Autodesk Inventor part; units mm, degrees
ref_plane "YZ Plane" through (0, 0, 0) normal (1, 0, 0) x (0, 1, 0)
ref_plane "XZ Plane" through (0, 0, 0) normal (0, 1, 0) x (-1, 0, 0)
ref_plane "XY Plane" through (0, 0, 0) normal (0, 0, 1) x (1, 0, 0)
sketch "Sketch1" plane through (0, 0, 0) normal (0, 0, 1) x (1, 0, 0)
  line L0 (-12.7, 12.7) -> (12.7, 12.7)
  line L1 (12.7, 12.7) -> (12.7, -12.7)
  line L2 (12.7, -12.7) -> (-12.7, -12.7)
  line L3 (-12.7, -12.7) -> (-12.7, 12.7)
  line L4 (0, 17.78) -> (0, -17.78)
  line L5 (-17.78, 0) -> (17.78, 0)
  line L6 (9.525, 9.525) -> (-9.525, 9.525)
  line L7 (-9.525, 9.525) -> (-9.525, -9.525)
  line L8 (-9.525, -9.525) -> (9.525, -9.525)
  line L9 (9.525, -9.525) -> (9.525, 9.525)
  point P0 (0, 0)
  dimension "d0" = 25.4
  dimension "d1" = 3.175
extrude "Extrusion1" add sketch "Sketch1" along normal mid plane 1502.0343 contours L0 L4 L6 L7 L5 L3 | L0 L1 L5 L9 L6 L4 | L5 L7 L8 L4 L2 L3 | L1 L2 L4 L8 L9 L5
sketch "Sketch2" plane through (12.7, 12.7, 751.0172) normal (1, 0, 0) x (0, 0, -1)
  line L0 (-300.4069, -12.7) -> (1802.4412, -12.7)
  line L1 (751.0172, -30.48) -> (751.0172, 5.08)
  circle A0 centre (12.7, -12.7) radius 3.175
  circle A1 centre (1489.3343, -12.7) radius 3.175
  point P0 (751.0172, -12.7)
  dimension "d4" = 1476.6343
  dimension "d5" = 6.35
extrude "Extrusion2" cut sketch "Sketch2" against normal up to surface (25.4 mm away)
equation "\"d2\" = Length"
equation "\"d6\" = Length"
properties part number "NTowerSupport" material "Aluminum 6061"
Input: part model. Units: mm. Frame: model coordinates. Give positions to 0.01 mm unless a question says otherwise; leave off trailing zeros. Order: outer loops, then holes, each group sorted by start corner. A loop starts at its lowest first (then second) coordinate and runs counter-clockwise, first axis right, second up. Notation, with made-up numbers: M 75,-38 L 113,-38 A16 ccw 113,-18 Z; hole C 78.25,-22.5 d3. An arc over 180 degrees is marked long. One line per question, with ' | ' between items.
1) Ray query, L1, parallel to X at y = 5.5, z = 561.5 (3 decimals); L2, parallel to Z at x = -11, y = 2. Return the intervals inside material, ascending.
Filled in:
L1: x = -12.7 to -9.525, 9.525 to 12.7 | L2: z = -751.02 to -740.78, -735.85 to 735.85, 740.78 to 751.02
2) Section B-B on z = -578.5. Output: boundary loops of the cut face in (x, y) (3 decimals).
Filled in:
outline: M -12.7,-12.7 L 12.7,-12.7 L 12.7,12.7 L -12.7,12.7 Z; hole M -9.525,-9.525 L 9.525,-9.525 L 9.525,9.525 L -9.525,9.525 Z
3) Section A-A on x = 2. Output: boundary loops of the cut face in (y, z) (3 decimals), and give its area (3 significant figures).
Filled in:
outline: M -12.7,-751.017 L -9.525,-751.017 L -9.525,751.017 L -12.7,751.017 Z; M 9.525,-751.017 L 12.7,-751.017 L 12.7,751.017 L 9.525,751.017 Z | area: 9,540 mm2
4) Contact query for a flat-ended pin moving along its axis: P1, Ø5, axis at y = 0, z = 738.32, coming from the -X side. Output: stop coordinate, or through.
Filled in:
P1: passes through
